Work out the finished part from the listing and answer in its coordinate system (mm). Coordinates: 2 decimals unless noted, no trailing zeros. Loops run counter-clockwise (first coordinate to the right, second up) from the corner with the lowest first, then second, coordinate; pieces in that order, holes last. Notation, with made-up numbers: (-3, 13) -> (19, 13) arc R33 ccw to (19, 41) -> close; hole circle Ø7 at (16.25, -16). An arc over 180 degrees is marked (long way). One line per question, with ' | ' between items.
```python
from build123d import *

# Parameters (mm, degrees)
SKETCH_1_W           = 220
SKETCH_1_H           = 220
SKETCH_1_R           = 1.6
EXTRUDE_1_DEPTH      = 6
EXTRUDE_2_DEPTH      = 20
EXTRUDE_2_DEPTH_BACK = 6
SKETCH_2_R           = 1.6


with BuildPart() as part:
    # 草图1 → 凸台-拉伸1 (new body)
    with BuildSketch(Plane(origin=(0, 0, 0), x_dir=(0, 0, -1), z_dir=(1, 0, 0))):
        with Locations((-23.204600907, 15.424234721)):
            Rectangle(SKETCH_1_W, SKETCH_1_H)
        with Locations((81.295399093, 119.924234721)):
            Circle(SKETCH_1_R, mode=Mode.SUBTRACT)
        with Locations((-127.704600907, 119.924234721)):
            Circle(SKETCH_1_R, mode=Mode.SUBTRACT)
        with Locations((-127.704600907, -89.075765279)):
            Circle(SKETCH_1_R, mode=Mode.SUBTRACT)
        with Locations((81.295399093, -89.075765279)):
            Circle(SKETCH_1_R, mode=Mode.SUBTRACT)
    extrude(amount=EXTRUDE_1_DEPTH)

    # 草图2 → 凸台-拉伸2 (add, two sides: drawn at the far end of the back side and taken through both)
    with BuildSketch(Plane(origin=(6, 0, 0), x_dir=(0, 0, -1), z_dir=(1, 0, 0)).offset(-EXTRUDE_2_DEPTH_BACK)):
        with Locations((81.295399093, -89.075765279)):
            Circle(SKETCH_2_R)
        with Locations((-127.704600907, -89.075765279)):
            Circle(SKETCH_2_R)
        with Locations((81.295399093, 119.924234721)):
            Circle(SKETCH_2_R)
        with Locations((-127.704600907, 119.924234721)):
            Circle(SKETCH_2_R)
    extrude(amount=EXTRUDE_2_DEPTH + EXTRUDE_2_DEPTH_BACK)


solid = part.part
```
1) Find section C-C (y = 26.5). Write down the section's boundary in (x, z).
Check values:
outline: (0, -86.8) -> (6, -86.8) -> (6, 133.2) -> (0, 133.2) -> close
2) A flat-ended cylindrical pin translates along its axis: pin 1 (6 mm diameter, centred on y = -65, z = -18.5, fed in from +X). Find the tip coordinate at first contact, or state that the pin passes through.
Check values:
pin 1: stops at x = 6
3) Find the intervals of material crossed by line 1 along X through (y, z) = (-31, -67), in increasing order.
Check values:
line 1: x = 0 to 6
4) Find section B-B (x = 18.25). Write down the section's boundary in (y, z).
Check values:
outline: circle Ø3.2 at (-89.08, -81.3); circle Ø3.2 at (-89.08, 127.7); circle Ø3.2 at (119.92, -81.3); circle Ø3.2 at (119.92, 127.7)
5) Find section A-A (z = -72). Write down the section's boundary in (x, y), plus the area to 3 significant figures.
Check values:
outline: (0, -94.58) -> (6, -94.58) -> (6, 125.42) -> (0, 125.42) -> close | area: 1,320 mm^2
